Verification items for the finished model (mm, model axes). Face numbers are marked on the shaded views. A direction names the side the tool comes from. Give positions to 0.01 mm unless a question says otherwise; leave off trailing zeros. Loops run counter-clockwise (first coordinate to the right, second up) from the corner with the lowest first, then second, coordinate; pieces in that order, holes last. Notation, with made-up numbers: M 0,56.5 L 31,56.5 A13 ccw 31,76.5 Z; hole C 42.25,53 d9. An arc over 180 degrees is marked long. Write each question's results on one line, items separated by ' | '. Start each with the question number.
```python
from build123d import *

# Parameters (mm, degrees)
SKETCH1_W           = 150
SKETCH1_H           = 18.7
BOSS_EXTRUDE1_DEPTH = 10
SKETCH2_R           = 3
CUT_EXTRUDE1_DEPTH  = 10
SKETCH3_R           = 0.9
CUT_EXTRUDE2_DEPTH  = 5
SKETCH4_W           = 10
SKETCH4_H           = 18.7
BOSS_EXTRUDE2_DEPTH = 80
SKETCH5_W           = 10
SKETCH5_H           = 24
CUT_EXTRUDE3_DEPTH  = 15.7
SKETCH6_W           = 10
SKETCH6_H           = 24
SKETCH6_W_2         = 5
BOSS_EXTRUDE3_DEPTH = 3
CHAMFER1_SIZE       = 10
CHAMFER2_SIZE       = 2
SKETCH7_W           = 10
SKETCH7_H           = 10
CUT_EXTRUDE4_DEPTH  = 3
SKETCH9_R           = 1.4
CUT_EXTRUDE5_DEPTH  = 10
CUT_EXTRUDE6_DEPTH  = 20
CHAMFER3_SIZE       = 5
CHAMFER4_SIZE       = 5
CHAMFER5_SIZE       = 3
SKETCH11_W          = 9
SKETCH11_H          = 3
CUT_EXTRUDE7_DEPTH  = 20
FILLET1_R           = 1
SKETCH12_W          = 3
SKETCH12_H          = 9
CUT_EXTRUDE8_DEPTH  = 20
FILLET2_R           = 1
SKETCH13_R          = 1.55
CUT_EXTRUDE9_DEPTH  = 20
SKETCH14_R          = 0.9
CUT_EXTRUDE10_DEPTH = 3
CHAMFER6_SIZE       = 2


with BuildPart() as part:
    # Sketch1 → Boss-Extrude1 (new body)
    with BuildSketch(Plane(origin=(0, 0, 0), x_dir=(1, 0, 0), z_dir=(0, 1, 0))):
        Rectangle(SKETCH1_W, SKETCH1_H)
    extrude(amount=BOSS_EXTRUDE1_DEPTH)

    # Sketch2 → Cut-Extrude1 (cut)
    with BuildSketch(Plane(origin=(0, 10, 0), x_dir=(1, 0, 0), z_dir=(0, 1, 0))):
        with Locations(Location((0, 0, 0), (0, 0, 270))):
            Circle(SKETCH2_R)
    extrude(amount=-CUT_EXTRUDE1_DEPTH, mode=Mode.SUBTRACT)

    # Sketch3 → Cut-Extrude2 (cut)
    with BuildSketch(Plane.XZ):
        with Locations(Location((7.25, 0, 0), (0, 0, 270))):
            Circle(SKETCH3_R)
        with Locations(Location((-7.25, 0, 0), (0, 0, 270))):
            Circle(SKETCH3_R)
    extrude(amount=-CUT_EXTRUDE2_DEPTH, mode=Mode.SUBTRACT)

    # Sketch4 → Boss-Extrude2 (add)
    with BuildSketch(Plane(origin=(0, 10, 0), x_dir=(1, 0, 0), z_dir=(0, 1, 0))):
        with Locations((-70, 0)):
            Rectangle(SKETCH4_W, SKETCH4_H)
        with Locations((70, 0)):
            Rectangle(SKETCH4_W, SKETCH4_H)
    extrude(amount=BOSS_EXTRUDE2_DEPTH)

    # Sketch5 → Cut-Extrude3 (cut)
    with BuildSketch(Plane.XY.offset(9.35)):
        with Locations((-70, 58)):
            Rectangle(SKETCH5_W, SKETCH5_H)
    extrude(amount=-CUT_EXTRUDE3_DEPTH, mode=Mode.SUBTRACT)

    # Sketch6 → Boss-Extrude3 (add)
    with BuildSketch(Plane.XY.offset(-6.35)):
        with Locations((-80, 58)):
            Rectangle(SKETCH6_W, SKETCH6_H)
        with Locations((-62.5, 58)):
            Rectangle(SKETCH6_W_2, SKETCH6_H)
    extrude(amount=-BOSS_EXTRUDE3_DEPTH)

    # Chamfer1
    # the kernel refuses this chamfer: 10 mm, written as the material it adds along each edge
    with BuildSketch(Plane(origin=(-75, 70, -6.35), x_dir=(0.027495876610586317, 0.9996219169112968, 0), z_dir=(0, 0, -1))) as chamfer1_piece_1:
        Polygon((CHAMFER1_SIZE * 0.999621916911, -CHAMFER1_SIZE * 0.0274958766106), (-CHAMFER1_SIZE * 0.0274958766106, -CHAMFER1_SIZE * 0.999621916911), (0, 0), align=None)
    extrude(amount=3)
    with BuildSketch(Plane(origin=(-75, 46, -6.35), x_dir=(0.027495876610586317, -0.9996219169112968, 0), z_dir=(0, 0, -1))) as chamfer1_piece_2:
        Polygon((CHAMFER1_SIZE * 0.999621916911, CHAMFER1_SIZE * 0.0274958766106), (-CHAMFER1_SIZE * 0.0274958766106, CHAMFER1_SIZE * 0.999621916911), (0, 0), align=None)
    extrude(amount=3)
    with BuildSketch(Plane(origin=(-65, 46, -6.35), x_dir=(-0.027495876610586317, -0.9996219169112968, 0), z_dir=(0, 0, -1))) as chamfer1_piece_3_section:
        Polygon((CHAMFER1_SIZE * 0.999621916911, -CHAMFER1_SIZE * 0.0274958766106), (-CHAMFER1_SIZE * 0.0274958766106, -CHAMFER1_SIZE * 0.999621916911), (0, 0), align=None)
    chamfer1_piece_3 = extrude(amount=3, mode=Mode.PRIVATE)
    chamfer1_piece_3 = split(chamfer1_piece_3, bisect_by=Plane(origin=(-60, 42.111111111, -7.85), z_dir=(-1, 0, 0)), keep=Keep.TOP, mode=Mode.PRIVATE)
    add(chamfer1_piece_3)
    with BuildSketch(Plane(origin=(-65, 70, -6.35), x_dir=(-0.027495876610586317, 0.9996219169112968, 0), z_dir=(0, 0, -1))) as chamfer1_piece_4_section:
        Polygon((CHAMFER1_SIZE * 0.999621916911, CHAMFER1_SIZE * 0.0274958766106), (-CHAMFER1_SIZE * 0.0274958766106, CHAMFER1_SIZE * 0.999621916911), (0, 0), align=None)
    chamfer1_piece_4 = extrude(amount=3, mode=Mode.PRIVATE)
    chamfer1_piece_4 = split(chamfer1_piece_4, bisect_by=Plane(origin=(-60, 73.888888889, -7.85), z_dir=(-1, 0, 0)), keep=Keep.TOP, mode=Mode.PRIVATE)
    add(chamfer1_piece_4)

    # Chamfer2
    chamfer2_edges = [part.edges().sort_by_distance(p)[0] for p in [
        (-75, 46, 1.5),
    ]]
    chamfer(chamfer2_edges, length=CHAMFER2_SIZE)

    # Sketch7 → Cut-Extrude4 (cut)
    with BuildSketch(Plane.XY.offset(9.35)):
        with Locations((-70, 75)):
            Rectangle(SKETCH7_W, SKETCH7_H)
        with Locations((-70, 41)):
            Rectangle(SKETCH7_W, SKETCH7_H)
    extrude(amount=-CUT_EXTRUDE4_DEPTH, mode=Mode.SUBTRACT)

    # Sketch9 → Cut-Extrude5 (cut)
    with BuildSketch(Plane.XY.offset(6.35)):
        with Locations((-70, 75)):
            Circle(SKETCH9_R)
        with Locations((-70, 41)):
            Circle(SKETCH9_R)
    extrude(amount=-CUT_EXTRUDE5_DEPTH, mode=Mode.SUBTRACT)

    # Sketch10 → Cut-Extrude6 (cut)
    with BuildSketch(Plane.XY.offset(9.35)):
        Polygon((65, 90), (75, 90), (75, 40), (72, 40), (72, 30), (68, 30), (68, 40), (65, 40), align=None)
    extrude(amount=-CUT_EXTRUDE6_DEPTH, mode=Mode.SUBTRACT)

    # Chamfer3
    chamfer3_edges = [part.edges().sort_by_distance(p)[0] for p in [
        (-75, 90, 0),
    ]]
    chamfer(chamfer3_edges, length=CHAMFER3_SIZE)

    # Chamfer4
    chamfer4_edges = [part.edges().sort_by_distance(p)[0] for p in [
        (-75, 0, 0),
        (75, 0, 0),
    ]]
    chamfer(chamfer4_edges, length=CHAMFER4_SIZE)

    # Chamfer5
    chamfer5_edges = [part.edges().sort_by_distance(p)[0] for p in [
        (-65, 10, 0),
        (65, 10, 0),
    ]]
    chamfer(chamfer5_edges, length=CHAMFER5_SIZE)

    # Sketch11 → Cut-Extrude7 (cut)
    with BuildSketch(Plane(origin=(0, 10, 0), x_dir=(1, 0, 0), z_dir=(0, 1, 0))):
        with Locations((-47.5, 0.450329583)):
            Rectangle(SKETCH11_W, SKETCH11_H)
    extrude(amount=-CUT_EXTRUDE7_DEPTH, mode=Mode.SUBTRACT)

    # Fillet1
    fillet1_edges = [part.edges().sort_by_distance(p)[0] for p in [
        (-43, 5, -1.950329583),
        (-43, 5, 1.049670417),
        (-52, 5, 1.049670417),
        (-52, 5, -1.950329583),
    ]]
    fillet(fillet1_edges, radius=FILLET1_R)

    # Sketch12 → Cut-Extrude8 (cut)
    with BuildSketch(Plane(origin=(-65, 0, 0), x_dir=(0, 0, -1), z_dir=(1, 0, 0))):
        with Locations((0, 19.5)):
            Rectangle(SKETCH12_W, SKETCH12_H)
    extrude(amount=-CUT_EXTRUDE8_DEPTH, mode=Mode.SUBTRACT)

    # Fillet2
    fillet2_edges = [part.edges().sort_by_distance(p)[0] for p in [
        (-70, 24, -1.5),
        (-70, 15, -1.5),
        (-70, 15, 1.5),
        (-70, 24, 1.5),
    ]]
    fillet(fillet2_edges, radius=FILLET2_R)

    # Sketch13 → Cut-Extrude9 (cut)
    with BuildSketch(Plane(origin=(75, 0, 0), x_dir=(0, 0, -1), z_dir=(1, 0, 0))):
        with Locations((0, 35)):
            Circle(SKETCH13_R)
    extrude(amount=-CUT_EXTRUDE9_DEPTH, mode=Mode.SUBTRACT)

    # Sketch14 → Cut-Extrude10 (cut)
    with BuildSketch(Plane(origin=(-65, 0, 0), x_dir=(0, 0, -1), z_dir=(1, 0, 0))):
        with Locations((0, 72.5)):
            Circle(SKETCH14_R)
        with Locations((0, 43.5)):
            Circle(SKETCH14_R)
    extrude(amount=-CUT_EXTRUDE10_DEPTH, mode=Mode.SUBTRACT)

    # Chamfer6
    chamfer6_edges = [part.edges().sort_by_distance(p)[0] for p in [
        (-75, 70, 0),
    ]]
    chamfer(chamfer6_edges, length=CHAMFER6_SIZE)


solid = part.part
```
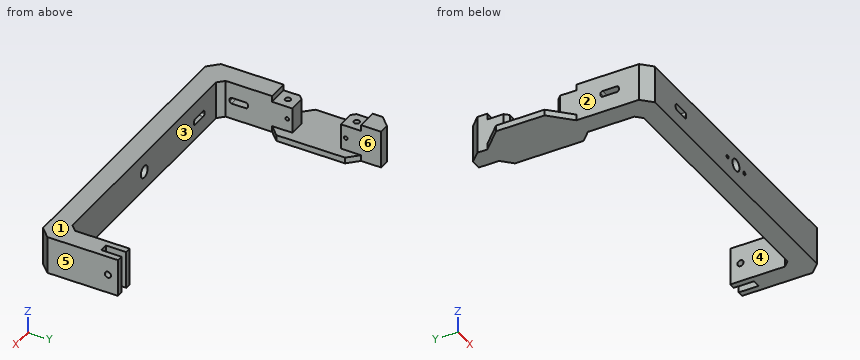
1. Release check for a two-part mould opening along X. For the marked faces 1, 2 and 3 record: released by +X, released by -X, zero draft, split by the parting line, or undercut.
2. Set-up check for the marked faces 4, 5 and 6: record each of +Z, -Z, +X, -X, +Y, -Y from which the full face is reachable in a straight line by a thin tool's end or side.
3. Thickness scan on probe 1 along Y at (x, z) = (-66.7, 0); probe 2 along X at (y, z) = (75, 2); probe 3 along X at (y, z) = (27, 1.25). Record the ranges inside material, lowest first.
4. Section check C-C, the plane x = 38. Record the boundary of the cut face in (y, z).
5. Section check B-B, the plane y = 48.5. Record the boundary of the cut face in (x, z), plus the area to 3 significant figures.
6. Section check A-A, the plane x = -47. Record the boundary of the cut face in (y, z), plus the area to 3 significant figures.
7. Depth check by flat-ended pin: pin 1 Ø1.5 at (x, z) = (-9, -4) entering from +Y; pin 2 Ø2.5 at (y, z) = (43.5, 0) entering from -X; pin 3 Ø0.9 at (y, z) = (66, -7.5) entering from +X. Enter the tip coordinate at first touch or a pass-through.
Filled sheet:
1) face 1: zero draft | face 2: released by -X | face 3: undercut
2) face 4: +Z, -Z, +Y | face 5: +Z, -Z, +X, +Y, -Y | face 6: +Z, +X, +Y
3) probe 1: 0 to 15, 24 to 42.6, 44.4 to 46, 70 to 71.6, 73.4 to 90 | probe 2: -75 to -71.4, -68.6 to -65 | probe 3: -75 to -65, 65 to 75
4) outline: M 0,-9.35 L 10,-9.35 L 10,9.35 L 0,9.35 Z
5) outline: M -85,-9.35 L -60,-9.35 L -60,-6.35 L -85,-6.35 Z | area: 75.0 mm2
6) outline: M 0,-9.35 L 10,-9.35 L 10,-1.95 L 0,-1.95 Z; M 0,1.05 L 10,1.05 L 10,9.35 L 0,9.35 Z | area: 157 mm2
7) pin 1: y = 10 | pin 2: x = -75 | pin 3: x = -60
